Could you check a few things on this model? Use its own coordinates, in mm. Face numbers are marked on the shaded views. Coordinates: 2 decimals unless noted, no trailing zeros. Loops run counter-clockwise (first coordinate to the right, second up) from the corner with the lowest first, then second, coordinate; pieces in that order, holes last.
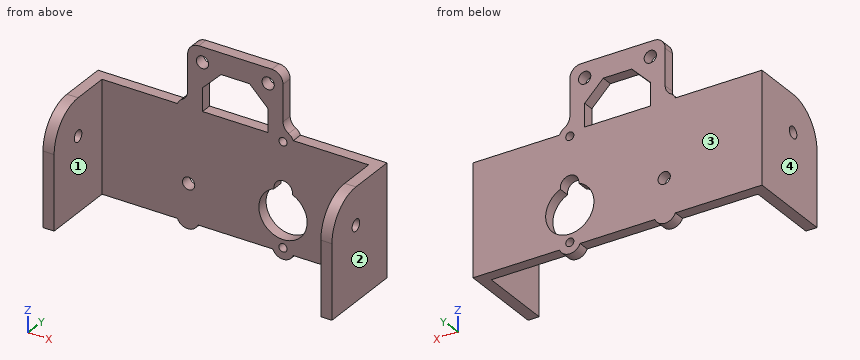
from build123d import *

# Parameters (mm, degrees)
SKETCH1_W           = 3
SKETCH1_H           = 20
SKETCH1_H_2         = 3
SKETCH1_W_2         = 71.840634077
BOSS_EXTRUDE1_DEPTH = 30
FILLET1_R           = 10
SKETCH2_R           = 1.575
CUT_EXTRUDE1_DEPTH  = 50
SKETCH3_R           = 6.5
SKETCH3_R_2         = 2.5
SKETCH3_R_3         = 1.1
SKETCH3_R_4         = 1.65
CUT_EXTRUDE2_DEPTH  = 3
SKETCH4_R           = 1.65
BOSS_EXTRUDE2_DEPTH = 3
FILLET3_R           = 3


with BuildPart() as part:
    # Sketch1 → Boss-Extrude1 (new body)
    with BuildSketch(Plane.XY):
        with Locations((-37.346255817, -2.476707935)):
            Rectangle(SKETCH1_W, SKETCH1_H)
        with Locations((-37.346255817, 9.023292065)):
            Rectangle(SKETCH1_W, SKETCH1_H_2)
        with Locations((0.074061222, 9.023292065)):
            Rectangle(SKETCH1_W_2, SKETCH1_H_2)
        with Locations((37.49437826, 9.023292065)):
            Rectangle(SKETCH1_W, SKETCH1_H_2)
        with Locations((37.49437826, -2.476707935)):
            Rectangle(SKETCH1_W, SKETCH1_H)
    extrude(amount=BOSS_EXTRUDE1_DEPTH)

    # Fillet1
    fillet1_edges = [part.edges().sort_by_distance(p)[0] for p in [
        (37.49437826, -12.476707935, 30),
        (-37.346255817, -12.476707935, 30),
    ]]
    fillet(fillet1_edges, radius=FILLET1_R)

    # Sketch2 → Cut-Extrude1 (cut, symmetric)
    with BuildSketch(Plane(origin=(0, 0, 0), x_dir=(0, 0, -1), z_dir=(1, 0, 0))):
        with Locations((-20, -2.476707935)):
            Circle(SKETCH2_R)
    extrude(amount=CUT_EXTRUDE1_DEPTH, both=True, mode=Mode.SUBTRACT)

    # Sketch3 → Cut-Extrude2 (cut)
    with BuildSketch(Plane(origin=(0, 10.523292065, 0), x_dir=(1, 0, 0), z_dir=(0, 1, 0))):
        with Locations((12.913568062, -9.80768247)):
            Circle(SKETCH3_R)
        with Locations((12.988568062, -16.167156082)):
            Circle(SKETCH3_R_2)
        with Locations(Location((12.913568062, -1.15768247, 0), (0, 0, 270))):
            Circle(SKETCH3_R_3)
        with Locations(Location((12.913568062, -28.85768247, 0), (0, 0, 270))):
            Circle(SKETCH3_R_3)
        with Locations(Location((-12.507980061, -10.050384435, 0), (0, 0, 270))):
            Circle(SKETCH3_R_4)
    extrude(amount=-CUT_EXTRUDE2_DEPTH, mode=Mode.SUBTRACT)

    # Sketch4 → Boss-Extrude2 (add)
    # profile 1 of 5: a face of its own
    with BuildSketch(Plane(origin=(0, 10.523292065, 0), x_dir=(1, 0, 0), z_dir=(0, 1, 0))):
        with BuildLine():
            Line((15.687574309, -30), (10.139561814, -30))
            ThreePointArc((10.139561814, -30), (11.244279679, -31.350367026), (12.913568062, -31.85768247))
            ThreePointArc((12.913568062, -31.85768247), (14.582856444, -31.350367026), (15.687574309, -30))
        make_face()
    # profile 2 of 5: a face of its own
    with BuildSketch(Plane(origin=(0, 10.523292065, 0), x_dir=(1, 0, 0), z_dir=(0, 1, 0))):
        with BuildLine():
            Line((10.145938878, 0), (15.681197245, 0))
            ThreePointArc((15.681197245, 0), (12.913568062, 1.84231753), (10.145938878, 0))
        make_face()
    # profile 3 of 5: a face of its own
    with BuildSketch(Plane(origin=(0, 10.523292065, 0), x_dir=(1, 0, 0), z_dir=(0, 1, 0))):
        with BuildLine():
            Line((-3.765445619, -41.20768247), (-8.765445619, -36.20768247))
            Line((-8.765445619, -36.20768247), (-8.765445619, -30))
            Line((-8.765445619, -30), (-9.991439371, -30))
            ThreePointArc((-9.991439371, -30), (-11.096157236, -31.350367026), (-12.765445619, -31.85768247))
            Line((-12.765445619, -31.85768247), (-12.765445619, -46.85768247))
            Line((-12.765445619, -46.85768247), (-6.765445619, -46.85768247))
            Line((-6.765445619, -46.85768247), (6.913568062, -46.85768247))
            Line((6.913568062, -46.85768247), (12.913568062, -46.85768247))
            Line((12.913568062, -46.85768247), (12.913568062, -31.85768247))
            ThreePointArc((12.913568062, -31.85768247), (11.244279679, -31.350367026), (10.139561814, -30))
            Line((10.139561814, -30), (8.913568062, -30))
            Line((8.913568062, -30), (8.913568062, -36.20768247))
            Line((8.913568062, -36.20768247), (3.913568062, -41.20768247))
            Line((3.913568062, -41.20768247), (-3.765445619, -41.20768247))
        make_face()
        with Locations(Location((-8.765445619, -42.85768247, 0), (0, 0, 270))):
            Circle(SKETCH4_R, mode=Mode.SUBTRACT)
        with Locations(Location((8.913568062, -42.85768247, 0), (0, 0, 270))):
            Circle(SKETCH4_R, mode=Mode.SUBTRACT)
    # profile 4 of 5: a face of its own
    with BuildSketch(Plane(origin=(0, 10.523292065, 0), x_dir=(1, 0, 0), z_dir=(0, 1, 0))):
        with BuildLine():
            ThreePointArc((-12.765445619, -31.85768247), (-11.096157236, -31.350367026), (-9.991439371, -30))
            Line((-9.991439371, -30), (-15.539451866, -30))
            ThreePointArc((-15.539451866, -30), (-14.434734002, -31.350367026), (-12.765445619, -31.85768247))
        make_face()
    # profile 5 of 5: a face of its own
    with BuildSketch(Plane(origin=(0, 10.523292065, 0), x_dir=(1, 0, 0), z_dir=(0, 1, 0))):
        with BuildLine():
            Line((-15.533074803, 0), (-9.997816435, 0))
            ThreePointArc((-9.997816435, 0), (-12.765445619, 1.84231753), (-15.533074803, 0))
        make_face()
    extrude(amount=-BOSS_EXTRUDE2_DEPTH)

    # Fillet3
    fillet3_edges = [part.edges().sort_by_distance(p)[0] for p in [
        (12.913568062, 9.023292065, 31.85768247),
        (12.913568062, 9.023292065, 46.85768247),
        (-12.765445619, 9.023292065, 46.85768247),
        (-12.765445619, 9.023292065, 31.85768247),
    ]]
    fillet(fillet3_edges, radius=FILLET3_R)


solid = part.part
(1) For pin 1 (1.5 mm diameter, centred on y = 9.5, z = 33.5, fed in from -X); pin 2 (3 mm diameter, centred on x = 22.5, y = 8, fed in from -Z); pin 3 (10.5 mm diameter, centred on x = -30.5, y = 5, fed in from +Z), each with a flat end and sliding along its axis, tell me the tip position at first contact or that it passes through.
Answers:
pin 1: stops at x = -13.06
pin 2: stops at z = 0
pin 3: stops at z = 30
(2) Imagine slicing it at B-B, the plane z = 1.5. Write out the boundary of the cut face in (x, y).
Answers:
outline: (-38.85, -12.48) - (-35.85, -12.48) - (-35.85, 7.52) - (11.87, 7.52) - (11.87, 10.52) - (-38.85, 10.52) - close; (13.96, 7.52) - (35.99, 7.52) - (35.99, -12.48) - (38.99, -12.48) - (38.99, 10.52) - (13.96, 10.52) - close
(3) Imagine slicing it at C-C, the plane y = 9. State how many separate pieces and enclosed holes the cut face has, and give its area (3 significant figures).
Answers:
separate pieces: 1
enclosed holes: 7
area: 2,440 mm2
(4) I need wall thicknesses on probe 1 along X at (y, z) = (-9, 17.5); probe 2 along Y at (x, z) = (22, 26.5). Which ranges of each line are inside material? Lowest first, please.
Answers:
probe 1: x = -38.85 to -35.85, 35.99 to 38.99
probe 2: y = 7.52 to 10.52
(5) Imagine slicing it at D-D, the plane x = -32. Write out the boundary of the cut face in (y, z), and give its area (3 significant figures).
Answers:
outline: (7.52, 0) - (10.52, 0) - (10.52, 30) - (7.52, 30) - close
area: 90.0 mm2
(6) We'd pull the mould along X, two halves only. Please class the marked faces 1, 2, 3 and 4: +X half, -X half, draft (parallel to the pull), parting line (faces both ways), or undercut.
Answers:
face 1: undercut
face 2: +X half
face 3: draft
face 4: -X half
(7) Imagine slicing it at A-A, the plane y = 4.5. Write out the boundary of the cut face in (x, z), and give its area (3 significant figures).
Answers:
outline: (-38.85, 0) - (-35.85, 0) - (-35.85, 30) - (-38.85, 30) - close; (35.99, 0) - (38.99, 0) - (38.99, 30) - (35.99, 30) - close
area: 180 mm2
